Read the model definition and answer for the solid it produces. Units are mm, in the model's axes. A direction names the side the tool comes from. Give positions to 0.01 mm unless a question says otherwise; leave off trailing zeros. Order: outer loops, then holes, each group sorted by start corner. A loop starts at its lowest first (then second) coordinate and runs counter-clockwise, first axis right, second up. Notation, with made-up numbers: (-13, 87) - (-1, 87) arc R23 cw to (-1, 120) - close; hole circle Ø7 at (71.5, -24). An arc over 180 degrees is marked (long way). Write each question's results on one line, items separated by ' | '.
from build123d import *

# Parameters (mm, degrees)
F0_R        = 11.05
F1_DEPTH    = 7
F2_R        = 15.35
F2_R_2      = 11.05
F3_DEPTH    = 7
F4_R        = 15.35
F4_R_2      = 11.05
F5_DEPTH    = 7
F6_T4_DEPTH = 72.7584417561
F6_T9_DEPTH = 72.8584149398


# Not quite as in the source:
# - a fillet or chamfer that OpenCascade refuses, or shapes differently, is made with other operations: its cross-section is extruded or revolved along the edge and cut away or added


with BuildPart() as f1:
    # F0 (on Top) → F1 (new body)
    with BuildSketch(Plane.XY):
        with BuildLine():
            ThreePointArc((10.1980390272, -11), (13.7471921753, -6.0012254829), (15, 0))
            ThreePointArc((15, 0), (13.7471921753, 6.0012254829), (10.1980390272, 11))
            ThreePointArc((10.1980390272, 11), (5.4772255751, 13.9642400438), (0, 15))
            ThreePointArc((0, 15), (-5.4772255751, 13.9642400438), (-10.1980390272, 11))
            ThreePointArc((-10.1980390272, 11), (-15, 0), (-10.1980390272, -11))
            ThreePointArc((-10.1980390272, -11), (-5.4772255751, -13.9642400438), (0, -15))
            ThreePointArc((0, -15), (5.4772255751, -13.9642400438), (10.1980390272, -11))
        make_face()
        Circle(F0_R, mode=Mode.SUBTRACT)
        with BuildLine():
            ThreePointArc((0, 15), (5.4772255751, 13.9642400438), (10.1980390272, 11))
            Line((10.1980390272, 11), (30, 11))
            Line((30, 11), (30, 15))
            Line((30, 15), (0, 15))
        make_face()
        with BuildLine():
            Line((30, -11), (10.1980390272, -11))
            ThreePointArc((10.1980390272, -11), (5.4772255751, -13.9642400438), (0, -15))
            Line((0, -15), (30, -15))
            Line((30, -15), (30, -11))
        make_face()
        with BuildLine():
            ThreePointArc((-10.1980390272, 11), (-5.4772255751, 13.9642400438), (0, 15))
            Line((0, 15), (-30, 15))
            Line((-30, 15), (-29.9866729691, 11))
            Line((-29.9866729691, 11), (-10.1980390272, 11))
        make_face()
        with BuildLine():
            Line((-30, -15), (0, -15))
            ThreePointArc((0, -15), (-5.4772255751, -13.9642400438), (-10.1980390272, -11))
            Line((-10.1980390272, -11), (-29.9866702422, -11))
            Line((-29.9866702422, -11), (-30, -15))
        make_face()
    extrude(amount=F1_DEPTH)

    # F2 (on face) → F3 (join)
    with BuildSketch(Plane(origin=(-29.9496808123, 0.0998054981, 0), x_dir=(-0.003332421, -0.9999944475, 0), z_dir=(-0.9999944475, 0.003332421, 0))):
        with Locations((0, 3.5)):
            Circle(F2_R)
        with Locations((0, 3.5)):
            Circle(F2_R_2, mode=Mode.SUBTRACT)
    extrude(amount=F3_DEPTH)

    # F4 (on face) → F5 (join)
    with BuildSketch(Plane.YZ.offset(30)):
        with Locations((0, 3.5)):
            Circle(F4_R)
        with Locations((0, 3.5)):
            Circle(F4_R_2, mode=Mode.SUBTRACT)
    extrude(amount=F5_DEPTH)

    # F6: chamfer of 5 on 4 edges, made by hand


with BuildPart() as f6_tool2:
    # F6_s3 → F6_t4 (new body)
    with BuildSketch(Plane.YZ.offset(30)):
        Polygon((10, 7), (15, 2), (15, 7), align=None)
    extrude(amount=-F6_T4_DEPTH)

    split(bisect_by=Plane(origin=(-29.9496808123, 0.0998054981, 0), x_dir=(0, 0, 1), z_dir=(0.9999944475, -0.003332421, 0)), keep=Keep.TOP)


with BuildPart() as f1_1:
    add(f1.part)

    # F6_t1: cut F6_tool2
    add(f6_tool2.part, mode=Mode.SUBTRACT)


with BuildPart() as f6_tool7:
    # F6_s8 → F6_t9 (new body)
    with BuildSketch(Plane.YZ.offset(-42.8584149398)):
        Polygon((-10, 7), (-15, 2), (-15, 7), align=None)
    extrude(amount=F6_T9_DEPTH)

    split(bisect_by=Plane(origin=(-29.9496808123, 0.0998054981, 0), x_dir=(0, 0, 1), z_dir=(0.9999944475, -0.003332421, 0)), keep=Keep.TOP)


with BuildPart() as f1_2:
    add(f1_1.part)

    # F6_t6: cut F6_tool7
    add(f6_tool7.part, mode=Mode.SUBTRACT)

    # F6_s11 → F6_t12 (revolve, cut)
    with BuildSketch(Plane.XY.offset(3.5)):
        Polygon((32, 15.35), (37, 10.35), (37, 15.35), align=None)
    revolve(axis=Axis((37, 0, 3.5), (1, 0, 0)), mode=Mode.SUBTRACT)

    # F6_s13 → F6_t14 (revolve, cut)
    with BuildSketch(Plane.XY.offset(3.5)):
        Polygon((-32.0008223689, -15.2434444286), (-36.9841325015, -10.2268100865), (-37.0007946063, -15.2267823238), align=None)
    revolve(axis=Axis((-36.9496419446, 0.1231324448, 3.5), (-0.9999944475, 0.003332421, 0)), mode=Mode.SUBTRACT)


solid = f1_2.part
(1) Each of these flat-tipped pins is pushed along its axis until it touches: pin 1 (1.8 mm diameter, centred on x = -22.5, z = 4, fed in from +Y); pin 2 (15 mm diameter, centred on y = 0, z = 11, fed in from -X) (3 decimals); pin 3 (0.6 mm diameter, centred on x = -9, z = 1, fed in from +Y); pin 4 (5 mm diameter, centred on x = 7.5, y = -2, fed in from +Z). Where does it stop, or does it pass through?
Conclusion:
pin 1: y = 13.9 | pin 2: x = -36.275 | pin 3: y = 15 | pin 4: through
(2) Consider probe 1 along Y at (x, z) = (0, 1.5); probe 2 along Z at (x, y) = (31.75, 0). Determine where each line is inside the solid, lowest interval first. Write a range as [from, to].
Conclusion:
probe 1: [-15, -11.05], [11.05, 15] | probe 2: [-11.85, -7.55], [14.55, 18.85]
(3) The mould has two halves that part along Z. Classify faces 1 (the face through (30, 1, 15)), 2 (the face through (-33.051, 1.549, 14.456)), 3 (the face through (12, 0, 7)): pulls with the +Z half, pulls with the -Z half, needs draft (parallel to the pull), parting line crosses it, or undercut.
Conclusion:
face 1: needs draft | face 2: undercut | face 3: pulls with the +Z half
(4) Section A-A (x = 21.5) is taken. Give the vertices of the cut face in (y, z).
Conclusion:
outline: (-15, 0) - (-11, 0) - (-11, 6) - (-15, 2) - close; (11, 0) - (15, 0) - (15, 2) - (11, 6) - close
(5) Section C-C (x = 0) is taken. Give the vertices of the cut face in (y, z), plus the area to 3 significant figures.
Conclusion:
outline: (-15, 0) - (-11.05, 0) - (-11.05, 5.95) - (-15, 2) - close; (11.05, 0) - (15, 0) - (15, 2) - (11.05, 5.95) - close | area: 31.4 mm^2
(6) Section D-D (y = -2.5) is taken. State how many separate pieces and enclosed holes the cut face has, plus the area to 3 significant figures.
Conclusion:
separate pieces: 6 | enclosed holes: 0 | area: 129 mm^2
(7) For faces 4 (the face through (6, 10, 0)), 5 (the face through (20, -11, 3)), 6 (the face through (0, -13, 4)), 7 (the face through (0, 13, 4)), 8 (the face through (0, 15, 1)), determine the directions among +Z, -Z, +X, -X, +Y, -Y from which every point of the face is accessible in a straight line to the end or side of a thin tool.
Conclusion:
face 4: -Z, +Y, -Y | face 5: +Z, -Z | face 6: +Z, -Y | face 7: +Z, +Y | face 8: +Z, -Z, +Y
